Could you check a few things on this model? Use its own coordinates, in mm. A direction names the side the tool comes from. Round coordinates to 2 decimals unless told otherwise and drop trailing zeros. Loops run counter-clockwise (first coordinate to the right, second up) from the corner with the lowest first, then second, coordinate; pieces in that order, holes last. Notation, with made-up numbers: M 43,-15 L 76,-15 A8 cw 76,-8 Z; hole C 74,29 d2. An arc over 180 degrees is marked long. Return JSON: item names as keys, results as strings. Group by question number.
```python
from build123d import *

# Parameters (mm, degrees)
F1_DEPTH    = 1.5875
F2_DEPTH    = 3.175
F3_R        = 3.17499
F4_R        = 0.79375
F5_R        = 0.508
F7_DEPTH    = 1.5
F8_T1_DEPTH = 5.5
F8_T3_DEPTH = 3.716990566
F8_T5_DEPTH = 4.3856191038


# Not quite as in the source:
# - a fillet or chamfer that OpenCascade refuses, or shapes differently, is made with other operations: its cross-section is extruded or revolved along the edge and cut away or added
# - a fillet or chamfer is up to 0.001 mm smaller than in the source, because OpenCascade refuses the exact size


with BuildPart() as f1:
    # F0 (on Top) → F1 (new body, symmetric)
    with BuildSketch(Plane.XY):
        with BuildLine():
            Line((3.175, 4.7625), (3.175, 7.9375))
            ThreePointArc((3.175, 7.9375), (0, 9.525), (-3.175, 7.9375))
            Line((-3.175, 7.9375), (-3.175, 4.7625))
            Line((-3.175, 4.7625), (-1.5875, 4.7625))
            Line((-1.5875, 4.7625), (-1.5875, 3.175))
            Line((-1.5875, 3.175), (1.5875, 3.175))
            Line((1.5875, 3.175), (1.5875, 4.7625))
            Line((1.5875, 4.7625), (3.175, 4.7625))
        make_face()
    extrude(amount=F1_DEPTH, both=True)

    # F0 (on Top) → F2 (join, symmetric)
    with BuildSketch(Plane.XY):
        Polygon((6.35, 3.175), (1.5875, 3.175), (-1.5875, 3.175), (-6.35, 3.175), (-6.35, 0), (6.35, 0), align=None)
    extrude(amount=F2_DEPTH, both=True)

    # F3 (radius 3.175 in the source; OpenCascade refuses exactly that, so slightly less here)
    f3_edges = [f1.edges().sort_by_distance(p)[0] for p in [
        (6.35, 3.175, 0),
        (-6.35, 3.175, 0),
    ]]
    fillet(f3_edges, radius=F3_R)

    # F4
    f4_edges = [f1.edges().sort_by_distance(p)[0] for p in [
        (0, 9.525, -1.5875),
        (0, 9.525, 1.5875),
        (3.175, 6.35, -1.5875),
        (3.175, 6.35, 1.5875),
        (-3.175, 6.35, -1.5875),
        (-3.175, 6.35, 1.5875),
        (3.175, 7.9375, 0),
        (-3.175, 7.9375, 0),
    ]]
    fillet(f4_edges, radius=F4_R)

    # F5
    f5_edges = [f1.edges().sort_by_distance(p)[0] for p in [
        (0, 3.175, -1.5875),
        (-1.5875, 3.175, 0),
        (0, 3.175, 1.5875),
        (1.5875, 3.175, 0),
        (1.5875, 3.96875, 1.5875),
        (1.5875, 3.96875, -1.5875),
        (-1.5875, 3.96875, -1.5875),
        (-1.5875, 3.96875, 1.5875),
        (2.942516, 4.7625, 1.355016),
        (-2.942516, 4.7625, -1.355016),
        (1.984375, 4.7625, -1.5875),
        (-1.984375, 4.7625, -1.5875),
        (2.942516, 4.7625, -1.355016),
        (3.175, 4.7625, 0),
        (1.984375, 4.7625, 1.5875),
        (-3.175, 4.7625, 0),
        (-2.942516, 4.7625, 1.355016),
        (-1.984375, 4.7625, 1.5875),
    ]]
    fillet(f5_edges, radius=F5_R)

    # F6 (on Right) → F7 (join, symmetric)
    with BuildSketch(Plane.YZ):
        Polygon((0, -1), (0, 1), (-3, 1), (-3, 2), (-3.75, 2), (-5, 0), (-5, -1), align=None)
    extrude(amount=F7_DEPTH, both=True)

    # F8: fillet of radius 0.5 on 4 edges, made by hand

    # F8_s2 → F8_t1 (cut)
    with BuildSketch(Plane.YZ.offset(-2.75)):
        with BuildLine():
            ThreePointArc((-4.5, -1), (-4.8535533906, -0.8535533906), (-5, -0.5))
            Line((-5, -0.5), (-5, -1))
            Line((-5, -1), (-4.5, -1))
        make_face()
        with BuildLine():
            ThreePointArc((-3, 1.5), (-3.1464466094, 1.8535533906), (-3.5, 2))
            Line((-3.5, 2), (-3, 2))
            Line((-3, 2), (-3, 1.5))
        make_face()
    extrude(amount=F8_T1_DEPTH, mode=Mode.SUBTRACT)

    # F8_s4 → F8_t3 (cut)
    with BuildSketch(Plane.YZ.offset(-1.858495283)):
        with BuildLine():
            ThreePointArc((-5, -0.1433981132), (-4.9806243731, -0.0055568567), (-4.923999152, 0.1216013568))
            Line((-4.923999152, 0.1216013568), (-5, 0))
            Line((-5, 0), (-5, -0.1433981132))
        make_face()
    extrude(amount=F8_T3_DEPTH, mode=Mode.SUBTRACT)

    # F8_s6 → F8_t5 (cut)
    with BuildSketch(Plane.YZ.offset(-2.1928095519)):
        with BuildLine():
            ThreePointArc((-3.4728761792, 2), (-3.7152604454, 1.9373212406), (-3.8968753312, 1.76499947))
            Line((-3.8968753312, 1.76499947), (-3.75, 2))
            Line((-3.75, 2), (-3.4728761792, 2))
        make_face()
    extrude(amount=F8_T5_DEPTH, mode=Mode.SUBTRACT)


solid = f1.part
```
1. We'd pull the mould along Y, two halves only. Please class faces 1 (the face through (5.395, 2.27, -0.044)), 2 (the face through (0, 2, -3.175)), 3 (the face through (2, 4.762, 0)): +Y half, -Y half, draft (parallel to the pull), parting line (faces both ways), or undercut.
2. I'm going to push flat-ended pins straight in: pin 1 Ø0.9 at (x, z) = (2, 0.5) entering from -Y; pin 2 Ø3 at (x, z) = (-1.5, 0) entering from -Y; pin 3 Ø4 at (x, y) = (1, 6.5) entering from -Z; pin 4 Ø1.7 at (y, z) = (6, 0) entering from -X (3 decimals). Where does each tip first touch, or does it pass through?
3. I need wall thicknesses on probe 1 along Z at (x, y) = (1, 8.5); probe 2 along Y at (x, z) = (-1.25, -2.5) (3 decimals); probe 3 along Z at (x, y) = (-1.25, -1.75). Which ranges of each line are inside material? Lowest first, please.
4. On a 3-axis mill with a long thin cutter (end or side, diameter ignored), from which of +Z, -Z, +X, -X, +Y, -Y can I reach the whole of each face in a straight line? I mean faces 4 (the face through (-3.175, 6, 0)), 5 (the face through (3.175, 6, 0)), 6 (the face through (1.588, 4, 0)). Say none if no direction works.
5. If we section it at C-C, the plane x = -5: Please give me the cut outline in (y, z) (3 decimals), then the cut area to 3 significant figures.
6. If we section it at B-B, the plane y = -1.5: Please give me the cut outline in (x, z), then the cut area to 3 significant figures.
Geometry results:
{
 "1": {"face 1": "+Y half", "face 2": "draft", "face 3": "undercut"},
 "2": {"pin 1": "y = 0", "pin 2": "y = -5", "pin 3": "z = -1.59", "pin 4": "x = -3.175"},
 "3": {"probe 1": "-1.59 to 1.59", "probe 2": "0 to 3.175", "probe 3": "-1 to 1"},
 "4": {"face 4": "+Z, -Z, -X, +Y", "face 5": "+Z, -Z, +X, +Y", "face 6": "+Z, -Z, +X"},
 "5": {"outline": "M 0,-3.175 L 2.598,-3.175 L 2.598,3.175 L 0,3.175 Z", "area": "16.5 mm^2"},
 "6": {"outline": "M -1.5,-1 L 1.5,-1 L 1.5,1 L -1.5,1 Z", "area": "6.00 mm^2"}
}
